```python
from build123d import *

# Parameters (mm, degrees)
SKETCH1_R           = 3.5
BOSS_EXTRUDE1_DEPTH = 30


with BuildPart() as part:
    # Sketch1 → Boss-Extrude1 (new body)
    with BuildSketch(Plane.XY):
        with BuildLine():
            ThreePointArc((33.272867256, 6.376341239), (36.505813953, 6.6433833), (38.894452917, 8.83830009))
            ThreePointArc((38.894452917, 8.83830009), (41.196992362, 9.982453047), (43.465909091, 11.19191192))
            Line((43.465909091, 11.19191192), (42.5, 12.943202766))
            ThreePointArc((42.5, 12.943202766), (41.006656684, 12.138237192), (39.498073317, 11.362208804))
            ThreePointArc((39.498073317, 11.362208804), (32.494186047, 15.80345107), (31.008619489, 7.644274532))
            ThreePointArc((31.008619489, 7.644274532), (0, 2), (-31.008619489, 7.644274532))
            ThreePointArc((-31.008619489, 7.644274532), (-32.494186047, 15.80345107), (-39.498073317, 11.362208804))
            ThreePointArc((-39.498073317, 11.362208804), (-41.006656684, 12.138237192), (-42.5, 12.943202766))
            Line((-42.5, 12.943202766), (-43.465909091, 11.19191192))
            ThreePointArc((-43.465909091, 11.19191192), (-41.196992362, 9.982453047), (-38.894452917, 8.83830009))
            ThreePointArc((-38.894452917, 8.83830009), (-36.505813953, 6.6433833), (-33.272867256, 6.376341239))
            ThreePointArc((-33.272867256, 6.376341239), (0, 0), (33.272867256, 6.376341239))
        make_face()
        with Locations((-34.5, 11.223417185)):
            Circle(SKETCH1_R, mode=Mode.SUBTRACT)
        with Locations((34.5, 11.223417185)):
            Circle(SKETCH1_R, mode=Mode.SUBTRACT)
    extrude(amount=BOSS_EXTRUDE1_DEPTH)


solid = part.part
```
Geometry: final body of the model. Coordinates: model frame, mm. Give positions to 0.01 mm unless a question says otherwise; leave off trailing zeros. Order: outer loops, then holes, each group sorted by start corner. A loop starts at its lowest first (then second) coordinate and runs counter-clockwise, first axis right, second up. Notation, with made-up numbers: (64, -10.5) -> (76, -10.5) arc R24 ccw to (76, 4.5) -> close; hole circle Ø7 at (-35, 54). An arc over 180 degrees is marked (long way). Write each question's results on one line, items separated by ' | '. Start each with the question number.
1) Line query: line 1 (Y direction, x = 34.5, z = 10.25); line 2 (X direction, y = 13.75, z = 8.75); line 3 (X direction, y = 8.75, z = 11). Output: solid intervals per line, ascending. Write a range as from..to.
2) First-contact query: pin 1 (5.5 mm diameter, centred on x = 34.5, y = 11.22, fed in from -Z); pin 2 (5 mm diameter, centred on x = -24.5, z = 14.5, fed in from +Y); pin 3 (4 mm diameter, centred on x = -16, z = 11.5, fed in from +Y); pin 4 (4 mm diameter, centred on x = 23.5, z = 27, fed in from +Y). Flat tips, straight axial feed; report the tip coordinate or a pass-through.
3) Section D-D (z = 15.5). Return loops of the section in (x, y), then the cut area to 3 significant figures.
4) Section A-A (x = 34.5). Return loops of the section in (y, z), then the cut area to 3 significant figures.
5) Draft query along Y for faces 1 (the cylindrical face through (33.741, 7.807, 14.79)), 2 (the flat face through (-0.2, 1.5, 30)), 3 (the cylindrical face through (-36.548, 6.662, 14.79)). Return one class per face: pulls with the +Y half, pulls with the -Y half, needs draft (parallel to the pull), parting line crosses it, or undercut.
6) Section C-C (y = 13.75). Return loops of the section in (x, z), then the cut area to 3 significant figures.
7) Section B-B (y = 2.75). Return loops of the section in (x, z).
Calculated:
1) line 1: 6.22..7.72, 14.72..16.22 | line 2: -38.81..-36.92, -32.08..-30.19, 30.19..32.08, 36.92..38.81 | line 3: -38.85..-36.98, -32.02..-30.15, 30.15..32.02, 36.98..38.85
2) pin 1: through | pin 2: y = 6.24 | pin 3: y = 3.86 | pin 4: y = 5.78
3) outline: (-43.47, 11.19) arc R90 ccw to (-38.89, 8.84) arc R5 ccw to (-33.27, 6.38) arc R90 ccw to (33.27, 6.38) arc R5 ccw to (38.89, 8.84) arc R90 ccw to (43.47, 11.19) -> (42.5, 12.94) arc R88 cw to (39.5, 11.36) arc R5 ccw (long way) to (31.01, 7.64) arc R88 cw to (-31.01, 7.64) arc R5 ccw (long way) to (-39.5, 11.36) arc R88 cw to (-42.5, 12.94) -> close; hole circle Ø7 at (-34.5, 11.22); hole circle Ø7 at (34.5, 11.22) | area: 228 mm2
4) outline: (6.22, 0) -> (7.72, 0) -> (7.72, 30) -> (6.22, 30) -> close; (14.72, 0) -> (16.22, 0) -> (16.22, 30) -> (14.72, 30) -> close | area: 90.0 mm2
5) face 1: undercut | face 2: needs draft | face 3: pulls with the -Y half
6) outline: (-38.81, 0) -> (-36.92, 0) -> (-36.92, 30) -> (-38.81, 30) -> close; (-32.08, 0) -> (-30.19, 0) -> (-30.19, 30) -> (-32.08, 30) -> close; (30.19, 0) -> (32.08, 0) -> (32.08, 30) -> (30.19, 30) -> close; (36.92, 0) -> (38.81, 0) -> (38.81, 30) -> (36.92, 30) -> close | area: 227 mm2
7) outline: (-22.08, 0) -> (-11.46, 0) -> (-11.46, 30) -> (-22.08, 30) -> close; (11.46, 0) -> (22.08, 0) -> (22.08, 30) -> (11.46, 30) -> close
